Design review of the part built by this model. Coordinates are the model's own, in mm. Coordinates: 2 decimals unless noted, no trailing zeros. Loops run counter-clockwise (first coordinate to the right, second up) from the corner with the lowest first, then second, coordinate; pieces in that order, holes last. Notation, with made-up numbers: M 56.5,60.25 L 75.5,60.25 A25 ccw 75.5,75.25 Z; hole C 75.25,53 d9. An arc over 180 degrees is marked long. Write item = value, one per line. Start each with the question number.
from build123d import *

# Parameters (mm, degrees)
SKETCH1_W           = 335
SKETCH1_H           = 150
BOSS_EXTRUDE1_DEPTH = 5
SKETCH2_R           = 5.625
CUT_EXTRUDE1_DEPTH  = 10


with BuildPart() as part:
    # Sketch1 → Boss-Extrude1 (new body)
    with BuildSketch(Plane(origin=(0, 0, 0), x_dir=(1, 0, 0), z_dir=(0, 1, 0))):
        Rectangle(SKETCH1_W, SKETCH1_H)
    extrude(amount=BOSS_EXTRUDE1_DEPTH)

    # Sketch2 → Cut-Extrude1 (cut)
    with BuildSketch(Plane(origin=(0, 5, 0), x_dir=(1, 0, 0), z_dir=(0, 1, 0))):
        with Locations(Location((138.025, 59.315, 0), (0, 0, 270))):
            Circle(SKETCH2_R)
        with Locations(Location((-57.465, 59.315, 0), (0, 0, 270))):
            Circle(SKETCH2_R)
        with BuildLine():
            Line((143.49, -26.69), (143.49, -43.69))
            ThreePointArc((143.49, -43.69), (137.99, -49.19), (132.49, -43.69))
            Line((132.49, -43.69), (132.49, -26.69))
            ThreePointArc((132.49, -26.69), (137.99, -21.19), (143.49, -26.69))
        make_face()
        with BuildLine():
            Line((-51.96, -26.69), (-51.96, -43.69))
            ThreePointArc((-51.96, -43.69), (-57.46, -49.19), (-62.96, -43.69))
            Line((-62.96, -43.69), (-62.96, -26.69))
            ThreePointArc((-62.96, -26.69), (-57.46, -21.19), (-51.96, -26.69))
        make_face()
    extrude(amount=-CUT_EXTRUDE1_DEPTH, mode=Mode.SUBTRACT)


solid = part.part
Q1. To check wall thickness, follow line 1 (X direction, y = 2.85, z = 44.5); line 2 (X direction, y = 0.5, z = -60.5). State the ranges of each line that lie inside material, in increasing order. Write a range as from..to.
Q2. Mouldability with a two-part tool opening along Z and no side actions: class faces 1 (the face through (138.272, 2.535, -64.935)), 2 (the face through (-2, 5, -1)), 3 (the face through (-60.888, 2.535, -63.779)) as released by +Z, released by -Z, zero draft, split by the parting line, or undercut.
Q3. Add section A-A on y = 3.1. State the section outline as (x, z) points (3 decimals).
Values follow:
q1.line_1 = -167.5..-62.9, -52.02..132.55, 143.43..167.5
q1.line_2 = -167.5..-62.96, -51.97..132.53, 143.52..167.5
q2.face_1 = undercut
q2.face_2 = zero draft
q2.face_3 = undercut
q3.outline = M -167.5,-75 L 167.5,-75 L 167.5,75 L -167.5,75 Z; hole C -57.465,-59.315 d11.25; hole M -62.96,26.69 A5.5 ccw -51.96,26.69 L -51.96,43.69 A5.5 ccw -62.96,43.69 Z; hole C 138.025,-59.315 d11.25; hole M 132.49,26.69 A5.5 ccw 143.49,26.69 L 143.49,43.69 A5.5 ccw 132.49,43.69 Z
